The listing builds one solid part. Answer for the finished solid, in the listing's coordinates (mm). A direction names the side the tool comes from. Give positions to 0.01 mm unless a question says otherwise; leave off trailing zeros. Order: outer loops, then holes, each group sorted by start corner. A loop starts at its lowest first (then second) coordinate and runs counter-clockwise, first axis right, second up. Notation, with made-up numbers: (60, -1.75) - (113, -1.75) arc R30 ccw to (113, 20.25) - close; hole circle Ø4 at (-2, 53). An arc over 180 degrees is marked (long way). Answer as a JSON object with one key per item and string values. Group by question number.
Q1. A cutting plane is placed at C-C, the plane y = -2.25. Give the vertices of the cut face in (x, z) (3 decimals).
Q2. A cutting plane is placed at B-B, the plane z = 4.65. Give the vertices of the cut face in (x, y) (1 decimal).
Q3. The mould has two halves that part along X. Classify faces 3 (the face through (16.264, -0.116, 1.377)), 4 (the face through (0, 0, 0)), 5 (the face through (-9.861, 4.465, 1.377)): released by +X, released by -X, zero draft, split by the parting line, or undercut.
Q4. Given pin 1 (2 mm diameter, centred on x = 14.605, y = 0, fed in from +Z); pin 2 (1.7 mm diameter, centred on x = -1, y = -1, fed in from +Z) (3 decimals), each flat-ended and moving along its own axis, determine where each tip first touches the part or whether it passes through.
Q5. A cutting plane is placed at D-D, the plane x = 3.5. Give the vertices of the cut face in (y, z).
Q6. Consider line 1 (Z direction, x = -12.5, y = -2.5); line 2 (Y direction, x = -20, z = 1.5); line 3 (Z direction, x = -1.5, y = -0.25) (3 decimals). Determine where each line is inside the solid, lowest interval first.
Q7. For faces 1 (the face through (2.726, 0.858, 4.592)), 2 (the face through (-13.724, -0.116, 1.377)), determine the directions among +Z, -Z, +X, -X, +Y, -Y from which every point of the face is accessible in a straight line to the end or side of a thin tool.
Q8. A cutting plane is placed at A-A, the plane z = 1.4. Count the separate pieces of the cut face and the enclosed holes in it, and give its area (3 significant figures).
from build123d import *

# Parameters (mm, degrees)
SKETCH1_W         = 45.974
SKETCH1_H         = 11.811
EXTRUDE1_DEPTH    = 5.969
SKETCH2_OUTSIDE_W = 57.542
SKETCH2_OUTSIDE_H = 23.379
SKETCH2_OUTSIDE_R = 4.8895
EXTRUDE2_DEPTH    = 3.175
SKETCH3_R         = 2.8575
EXTRUDE3_DEPTH    = 2.794
LPATTERN1_COUNT   = 4
LPATTERN1_PITCH   = 2.54
EXTRUDE4_DEPTH    = 6.969


with BuildPart() as part:
    # Sketch1 → Extrude1 (new body)
    with BuildSketch(Plane.XY):
        Rectangle(SKETCH1_W, SKETCH1_H)
    extrude(amount=EXTRUDE1_DEPTH)

    # Sketch2 outside → Extrude2 (cut)
    with BuildSketch(Plane.XY.offset(5.969)):
        with Locations((0, -0.0005)):
            Rectangle(SKETCH2_OUTSIDE_W, SKETCH2_OUTSIDE_H)
        Circle(SKETCH2_OUTSIDE_R, mode=Mode.SUBTRACT)
    extrude(amount=-EXTRUDE2_DEPTH, mode=Mode.SUBTRACT)

    # Sketch3 → Extrude3 (cut)
    with BuildSketch(Plane.XY.offset(5.969)):
        Circle(SKETCH3_R)
    extrude(amount=-EXTRUDE3_DEPTH, mode=Mode.SUBTRACT)

    # Sketch5 → #50 (0.07) Diameter Hole1 (revolve, cut)
    with BuildSketch(Plane.YZ.offset(12.065)):
        Polygon((0, 0), (0, 5.61416509), (0.889, 5.08), (0.889, 0), align=None)
    f_50_0_07_diameter_hole1 = revolve(axis=Axis((12.065, 0, -6.35), (0, 0, 1)), mode=Mode.SUBTRACT)

    # LPattern1: #50 (0.07) Diameter Hole1 ×4
    with Locations(*[(i * LPATTERN1_PITCH, 0, 0) for i in range(1, LPATTERN1_COUNT)]):
        add(f_50_0_07_diameter_hole1, mode=Mode.SUBTRACT)

    # Mirror1: #50 (0.07) Diameter Hole1 across plane
    add(f_50_0_07_diameter_hole1.mirror(Plane(origin=(0, 0, 0), x_dir=(0, 0, 1), z_dir=(1, 0, 0))), mode=Mode.SUBTRACT)

    # Mirror1 copy 1 sketch → Mirror1 copy 1 (revolve, cut)
    with BuildSketch(Plane(origin=(-14.605, 0, 0), x_dir=(0, 1, 0), z_dir=(-1, 0, 0))):
        Polygon((0, 0), (0, -5.61416509), (0.889, -5.08), (0.889, 0), align=None)
    revolve(axis=Axis((-14.605, 0, -6.35), (0, 0, -1)), mode=Mode.SUBTRACT)

    # Mirror1 copy 2 sketch → Mirror1 copy 2 (revolve, cut)
    with BuildSketch(Plane(origin=(-17.145, 0, 0), x_dir=(0, 1, 0), z_dir=(-1, 0, 0))):
        Polygon((0, 0), (0, -5.61416509), (0.889, -5.08), (0.889, 0), align=None)
    revolve(axis=Axis((-17.145, 0, -6.35), (0, 0, -1)), mode=Mode.SUBTRACT)

    # Mirror1 copy 3 sketch → Mirror1 copy 3 (revolve, cut)
    with BuildSketch(Plane(origin=(-19.685, 0, 0), x_dir=(0, 1, 0), z_dir=(-1, 0, 0))):
        Polygon((0, 0), (0, -5.61416509), (0.889, -5.08), (0.889, 0), align=None)
    revolve(axis=Axis((-19.685, 0, -6.35), (0, 0, -1)), mode=Mode.SUBTRACT)

    # Sketch6 → Extrude4 (cut, through all)
    with BuildSketch(Plane(origin=(0, 0, 0), x_dir=(-1, 0, 0), z_dir=(0, 0, -1))):
        with BuildLine():
            Line((-61.04017999, 14.819304062), (0, 5.9055))
            Line((0, 5.9055), (20.0025, 2.9845))
            ThreePointArc((20.0025, 2.9845), (22.112860188, 2.110360188), (22.987, 0))
            ThreePointArc((22.987, 0), (22.112860188, -2.110360188), (20.0025, -2.9845))
            Line((20.0025, -2.9845), (0, -5.9055))
            Line((0, -5.9055), (-61.04017999, -14.819304062))
            Line((-61.04017999, -14.819304062), (62.335011618, -14.819304062))
            Line((62.335011618, -14.819304062), (62.335011618, 14.819304062))
            Line((62.335011618, 14.819304062), (-61.04017999, 14.819304062))
        make_face()
    extrude4 = extrude(amount=-EXTRUDE4_DEPTH, mode=Mode.SUBTRACT)

    # Mirror2: Extrude4 across plane
    add(extrude4.mirror(Plane(origin=(0, 0, 0), x_dir=(0, 0, 1), z_dir=(1, 0, 0))), mode=Mode.SUBTRACT)


solid = part.part
Reply:
{
 "1": {"outline": "(-21.963, 0) - (21.963, 0) - (21.963, 2.794) - (4.341, 2.794) - (4.341, 5.969) - (1.761, 5.969) - (1.761, 3.175) - (-1.761, 3.175) - (-1.761, 5.969) - (-4.341, 5.969) - (-4.341, 2.794) - (-21.963, 2.794) - close"},
 "2": {"outline": "circle Ø9.8 at (0, 0); hole circle Ø5.7 at (0, 0)"},
 "3": {"face 3": "undercut", "face 4": "zero draft", "face 5": "released by -X"},
 "4": {"pin 1": "stops at z = 2.79", "pin 2": "stops at z = 3.175"},
 "5": {"outline": "(-5.39, 0) - (5.39, 0) - (5.39, 2.79) - (3.41, 2.79) - (3.41, 5.97) - (-3.41, 5.97) - (-3.41, 2.79) - (-5.39, 2.79) - close"},
 "6": {"line 1": "z = 0 to 2.79", "line 2": "y = -2.98 to -0.83, 0.83 to 2.98", "line 3": "z = 0 to 3.175"},
 "7": {"face 1": "+Z", "face 2": "+Z, -Z"},
 "8": {"separate pieces": "1", "enclosed holes": "8", "area": "364 mm^2"}
}
